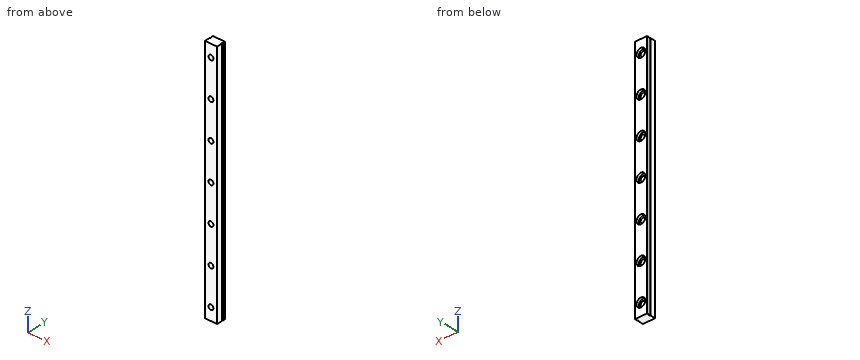
from build123d import *

# Parameters (mm, degrees)
BOSS_EXTRUDE1_DEPTH = 50
SKETCH2_R           = 1.8
CUT_EXTRUDE1_DEPTH  = 1
SKETCH3_R           = 1
CUT_EXTRUDE3_DEPTH  = 51.199003974
LPATTERN1_COUNT     = 7
LPATTERN1_PITCH     = 15
LPATTERN2_COUNT     = 7
LPATTERN2_PITCH     = 15


with BuildPart() as part:
    # Sketch1 → Boss-Extrude1 (new, symmetric)
    with BuildSketch(Plane.XY):
        with BuildLine():
            Line((-2.5, 3.7), (2.5, 3.7))
            Line((2.5, 3.7), (2.5, 2.7))
            ThreePointArc((2.5, 2.7), (2.25, 2.45), (2.5, 2.2))
            Line((2.5, 2.2), (2.5, 0))
            Line((2.5, 0), (-2.5, 0))
            Line((-2.5, 0), (-2.5, 2.2))
            ThreePointArc((-2.5, 2.2), (-2.25, 2.45), (-2.5, 2.7))
            Line((-2.5, 2.7), (-2.5, 3.7))
        make_face()
    extrude(amount=BOSS_EXTRUDE1_DEPTH, both=True)

    # Sketch2 → Cut-Extrude1 (cut)
    with BuildSketch(Plane(origin=(0, 3.7, 0), x_dir=(1, 0, 0), z_dir=(0, 1, 0))):
        with Locations(Location((0, 0, 0), (0, 0, 180))):
            Circle(SKETCH2_R)
    cut_extrude1 = extrude(amount=-CUT_EXTRUDE1_DEPTH, mode=Mode.SUBTRACT)

    # Sketch3 → Cut-Extrude3 (cut, through all)
    with BuildSketch(Plane(origin=(0, 3.7, 0), x_dir=(1, 0, 0), z_dir=(0, 1, 0))):
        with Locations(Location((0, 0, 0), (0, 0, 180))):
            Circle(SKETCH3_R)
    cut_extrude3 = extrude(amount=-CUT_EXTRUDE3_DEPTH, mode=Mode.SUBTRACT)

    # LPattern1: Cut-Extrude1, Cut-Extrude3 ×7
    with Locations(*[(0, 0, -i * LPATTERN1_PITCH) for i in range(1, LPATTERN1_COUNT)]):
        add(cut_extrude1, mode=Mode.SUBTRACT)
        add(cut_extrude3, mode=Mode.SUBTRACT)

    # LPattern2: Cut-Extrude1, Cut-Extrude3 ×7
    with Locations(*[(0, 0, i * LPATTERN2_PITCH) for i in range(1, LPATTERN2_COUNT)]):
        add(cut_extrude1, mode=Mode.SUBTRACT)
        add(cut_extrude3, mode=Mode.SUBTRACT)


solid = part.part
Build history of the part. All positions in model axes, mm. Give positions to 0.01 mm unless a question says otherwise; leave off trailing zeros. Loops run counter-clockwise (first coordinate to the right, second up) from the corner with the lowest first, then second, coordinate; pieces in that order, holes last. Notation, with made-up numbers: (-30, -34.5) -> (29, -34.5) arc R7 cw to (29, -30.5) -> close; hole circle Ø3 at (-0.75, 62). An arc over 180 degrees is marked (long way). Answer in a Markdown table with one row per item.
Item 1: Slice it at B-B on x = 0. Give the number of separate pieces and of enclosed holes in the cut face, plus the area to 3 significant figures.
Findings below:
| item | result |
|---|---|
| separate pieces | 8 |
| enclosed holes | 0 |
| area | 307 mm² |
Item 2: Slice it at A-A on z = 15. Write the cut outline in (x, y), plus the area to 3 significant figures.
Findings below:
| item | result |
|---|---|
| outline | (-2.5, 0) -> (-1, 0) -> (-1, 2.7) -> (-1.8, 2.7) -> (-1.8, 3.7) -> (-2.5, 3.7) -> (-2.5, 2.7) arc R0.25 cw to (-2.5, 2.2) -> close; (1, 0) -> (2.5, 0) -> (2.5, 2.2) arc R0.25 cw to (2.5, 2.7) -> (2.5, 3.7) -> (1.8, 3.7) -> (1.8, 2.7) -> (1, 2.7) -> close |
| area | 9.30 mm² |
Item 3: Flat gauge pin, fed straight in: P1, Ø2.5, axis at x = 0, z = 30, coming from the +Y side. Where does the tip first touch, or does it go through?
Findings below:
| item | result |
|---|---|
| P1 | stops at y = 2.7 |
Item 4: Probe line 1 along X through (y, z) = (2.4, 33.5); line 2 along Y through (x, z) = (2.35, 23). List the from-to ranges inside material, lowest first. Write a range as [from, to].
Findings below:
| item | result |
|---|---|
| line 1 | x = [-2.26, 2.26] |
| line 2 | y = [0, 2.25], [2.65, 3.7] |
